Autodesk Inventor part; units mm, degrees
ref_plane "YZ Plane" through (0, 0, 0) normal (1, 0, 0) x (0, 1, 0)
ref_plane "XZ Plane" through (0, 0, 0) normal (0, 1, 0) x (-1, 0, 0)
ref_plane "XY Plane" through (0, 0, 0) normal (0, 0, 1) x (1, 0, 0)
sketch "Sketch2" plane through (0, 0, 0) normal (1, 0, 0) x (0, 1, 0)
  line L0 (0, 0) -> (12, 0) construction
  line L1 (12, 0) -> (12, -5)
  line L2 (12, -5) -> (22, -10.7735)
  line L3 (22, -10.7735) -> (22, -13.5)
  line L4 (22, -13.5) -> (0, -13.5)
  line L5 (0, -13.5) -> (0, 0)
  line L6 (12, 0) -> (12, 5)
  line L7 (12, 5) -> (22, 10.7735)
  line L8 (22, 10.7735) -> (22, 13.5)
  line L9 (22, 13.5) -> (0, 13.5)
  line L10 (0, 13.5) -> (0, 0)
  line L11 (0, 0) -> (0, -46.5785) construction
  line L12 (22, -13.5) -> (22, -23.5)
  line L13 (22, -23.5) -> (0, -23.5)
  line L14 (0, -13.5) -> (0, -23.5)
  dimension "d0" = 22
  dimension "d1" = 13.5
  dimension "d2" = 5
  dimension "d3" = 60
  dimension "d4" = 10
  dimension "d16" = 10
revolve "Revolution1" add sketch "Sketch2" angle 360 about axis through (0, 0, 0) along (0, 0, -1)
sketch "Sketch3" plane through (0, 0, 13.5) normal (0, 0, 1) x (1, 0, 0)
  circle A0 centre (0, 0) radius 6
  line L0 (-2, 7.5) -> (2, 7.5)
  line L1 (2, 7.5) -> (2, 1.4561)
  line L2 (2, 1.4561) -> (-2, 1.4561)
  line L3 (-2, 1.4561) -> (-2, 7.5)
  line L4 (-2, 7.5) -> (2, 1.4561) construction
  line L5 (2, 7.5) -> (-2, 1.4561) construction
  line L6 (-5.2122, 6) -> (6.1572, 6) construction
  point P0 (0, 4.4781)
  point P1 (-2, 5.6569)
  point P2 (2, 5.6569)
  dimension "d6" = 12
  dimension "d7" = 4
  dimension "d9" = 1.5
extrude "Extrusion1" cut sketch "Sketch3" against normal through all
sketch "Sketch4" plane through (0, 0, -23.5) normal (0, 0, 1) x (1, 0, 0)
  circle A0 centre (0, -17) radius 3
  arc A1 (-2, 5.6569) -> (2, 5.6569) centre (0, 0) ccw construction
  line L0 (0, 0) -> (0, -6) construction
  line L1 (0, -6) -> (0, -17) construction
  line L2 (0, -17) -> (0, -25) construction
  circle A2 centre (0, 0) radius 25 construction
  dimension "d12" = 6
  dimension "d17" = 8
extrude "Extrusion2" cut sketch "Sketch4" along normal blind 10
properties part number "Vbelt Slave Pulley"
The model under review builds one solid part; all positions refer to its coordinate system, in mm. A direction names the side the tool comes from. Give positions to 0.01 mm unless a question says otherwise; leave off trailing zeros. Order: outer loops, then holes, each group sorted by start corner. A loop starts at its lowest first (then second) coordinate and runs counter-clockwise, first axis right, second up. Notation, with made-up numbers: (-3, 88) - (14, 88) arc R26 ccw to (14, 117) - close; hole circle Ø1 at (46.25, 41.5). An arc over 180 degrees is marked (long way). Use CSV: the item, a comma, the result in double quotes. Start each with the question number.
Q1. We need section C-C, the plane z = 4. Write out the cut boundary in (x, y).
Q2. Tool access review of faces 1 (the flat face through (-5, 5, 13.5)), 2 (the flat face through (0, 7.5, -5)), 3 (the flat face through (0, -17, -13.5)), 4 (the conical face through (12.52, -1.64, -5.36)): name each direction out of +Z, -Z, +X, -X, +Y, -Y from which nothing blocks a thin tool from reaching the whole face with its end or side.
Q3. To check wall thickness, follow line 1 along X through (y, z) = (5, -7); line 2 along Z through (x, y) = (17, -2.5); line 3 along Y through (x, z) = (-2.5, 5.5). State the ranges of each line that lie inside material, in increasing order. Write a range as [from, to].
Q4. We need section B-B, the plane x = 0. Write out the cut boundary in (y, z).
Q5. We need section D-D, the plane z = -19. Write out the cut boundary in (x, y), and give its area (3 significant figures).
Q6. The part is to be moulded in two halves that separate along Y. For faces 5 (the flat face through (-5, 5, -23.5)), 6 (the flat face through (-2, 7, -5)), 7 (the cylindrical face through (-21.477, -4.769, -17.226)), say which applies: +Y half, -Y half, draft (parallel to the pull), parting line (faces both ways), or undercut.
Q7. Clearance check with flat-ended pins moving along their axes: pin 1 Ø2 at (x, z) = (7, 1) entering from -Y; pin 2 Ø4 at (y, z) = (1.5, -6.5) entering from -X; pin 3 Ø1.5 at (y, z) = (7, -2.5) entering from -X. State where each tip first meets the part, or that it passes through.
Q8. We need section A-A, the plane y = 0. Write out the cut boundary in (x, z), and give its area (3 significant figures).
Outcome:
1,outline,"circle Ø24 at (0, 0); hole (-2, 5.66) arc R6 ccw (long way) to (2, 5.66) - (2, 7.5) - (-2, 7.5) - close"
2,face 1,"+Z, +X, -X, +Y, -Y"
2,face 2,"+Z, -Z"
2,face 3,"-Z"
2,face 4,"none"
3,line 1,"x = [-14.63, -3.32], [3.32, 14.63]"
3,line 2,"z = [-23.5, -7.99], [7.99, 13.5]"
3,line 3,"y = [-12.62, -5.45], [5.45, 12.62]"
4,outline,"(-22, -23.5) - (-20, -23.5) - (-20, -13.5) - (-14, -13.5) - (-14, -23.5) - (-6, -23.5) - (-6, 13.5) - (-22, 13.5) - (-22, 10.77) - (-12, 5) - (-12, -5) - (-22, -10.77) - close; (7.5, -23.5) - (22, -23.5) - (22, -10.77) - (12, -5) - (12, 5) - (22, 10.77) - (22, 13.5) - (7.5, 13.5) - close"
5,outline,"circle Ø44 at (0, 0); hole circle Ø6 at (0, -17); hole (-2, 5.66) arc R6 ccw (long way) to (2, 5.66) - (2, 7.5) - (-2, 7.5) - close"
5,area,"1,370 mm^2"
6,face 5,"draft"
6,face 6,"undercut"
6,face 7,"parting line"
7,pin 1,"stops at y = -10.39"
7,pin 2,"stops at x = -18"
7,pin 3,"stops at x = -10.24"
8,outline,"(-22, -23.5) - (-6, -23.5) - (-6, 13.5) - (-22, 13.5) - (-22, 10.77) - (-12, 5) - (-12, -5) - (-22, -10.77) - close; (6, -23.5) - (22, -23.5) - (22, -10.77) - (12, -5) - (12, 5) - (22, 10.77) - (22, 13.5) - (6, 13.5) - close"
8,area,"869 mm^2"
